from build123d import *

# Parameters (mm, degrees)
SKETCH1_W                        = 71
SKETCH1_H                        = 54
BOSS_EXTRUDE1_DEPTH              = 3.75
FILLET1_R                        = 1
SKETCH2_R                        = 7
CUT_EXTRUDE1_DEPTH               = 1
FILLET2_R                        = 0.25
SKETCH3_R                        = 0.5
CUT_EXTRUDE2_DEPTH               = 0.1
FILLET3_R                        = 0.25
M2_5_CLEARANCE_HOLE1_D           = 2.9
M2_5_CLEARANCE_HOLE1_DEPTH       = 1
M2_5_CLEARANCE_HOLE1_CSINK_D     = 2.95
M2_5_CLEARANCE_HOLE1_CSINK_ANGLE = 90
M2_5_CLEARANCE_HOLE1_TIP         = 0.871247898
M1_6_CLEARANCE_HOLE1_D           = 1


with BuildPart() as part:
    # Sketch1 → Boss-Extrude1 (new body)
    with BuildSketch(Plane.XY):
        Rectangle(SKETCH1_W, SKETCH1_H)
    extrude(amount=BOSS_EXTRUDE1_DEPTH)

    # Fillet1
    fillet1_edges = [part.edges().sort_by_distance(p)[0] for p in [
        (35.5, -27, 1.875),
        (-35.5, -27, 1.875),
        (-35.5, 27, 1.875),
        (35.5, 27, 1.875),
    ]]
    fillet(fillet1_edges, radius=FILLET1_R)

    # Sketch2 → Cut-Extrude1 (cut)
    with BuildSketch(Plane.XY.offset(3.75)):
        with BuildLine():
            Line((-34, -0.5), (-34, 17))
            Line((-34, 17), (-26.5, 24.5))
            Line((-26.5, 24.5), (-9, 24.5))
            ThreePointArc((-9, 24.5), (8.67766953, -18.17766953), (-34, -0.5))
        make_face()
        with Locations((-9, -0.5)):
            Circle(SKETCH2_R, mode=Mode.SUBTRACT)
    extrude(amount=-CUT_EXTRUDE1_DEPTH, mode=Mode.SUBTRACT)

    # Fillet2
    fillet2_edges = [part.edges().sort_by_distance(p)[0] for p in [
        (-16, -0.5, 3.75),
    ]]
    fillet(fillet2_edges, radius=FILLET2_R)

    # Sketch3 → Cut-Extrude2 (cut)
    with BuildSketch(Plane.XY.offset(3.75)):
        with Locations((-9, 4.1)):
            Circle(SKETCH3_R)
        with Locations((-12.983716857, 1.8)):
            Circle(SKETCH3_R)
        with Locations((-12.983716857, -2.8)):
            Circle(SKETCH3_R)
        with Locations((-9, -5.1)):
            Circle(SKETCH3_R)
        with Locations((-5.016283143, -2.8)):
            Circle(SKETCH3_R)
        with Locations((-5.016283143, 1.8)):
            Circle(SKETCH3_R)
    extrude(amount=-CUT_EXTRUDE2_DEPTH, mode=Mode.SUBTRACT)

    # Fillet3
    fillet3_edges = [part.edges().sort_by_distance(p)[0] for p in [
        (8.67766953, -18.17766953, 2.75),
        (-34, 8.25, 2.75),
        (-30.25, 20.75, 2.75),
        (-34, 17, 3.25),
        (-17.75, 24.5, 2.75),
        (-26.5, 24.5, 3.25),
        (-16, -0.5, 2.75),
        (8.67766953, -18.17766953, 3.75),
        (-17.75, 24.5, 3.75),
        (-30.25, 20.75, 3.75),
        (-34, 8.25, 3.75),
    ]]
    fillet(fillet3_edges, radius=FILLET3_R)

    # M2.5 Clearance Hole1
    with Locations(Plane.XY.offset(3.75)):
        with Locations((-9, -0.5)):
            CounterSinkHole(M2_5_CLEARANCE_HOLE1_D / 2, M2_5_CLEARANCE_HOLE1_CSINK_D / 2, depth=M2_5_CLEARANCE_HOLE1_DEPTH, counter_sink_angle=M2_5_CLEARANCE_HOLE1_CSINK_ANGLE)
            with Locations((0, 0, -(M2_5_CLEARANCE_HOLE1_DEPTH + M2_5_CLEARANCE_HOLE1_TIP / 2))):  # 118° drill point
                Cone(0, M2_5_CLEARANCE_HOLE1_D / 2, M2_5_CLEARANCE_HOLE1_TIP, mode=Mode.SUBTRACT)

    # M1.6 Clearance Hole1 (through all)
    with Locations(Plane.XY.offset(3.75)):
        with Locations((-169.780661566, 67.45785255), (-33.5, 22), (-30.6, 25), (3.1, 25), (33.5, 25), (8.2, 23.4), (33.5, -25), (3.1, -25), (-26.5, -21.5), (-29, -20), (-33.5, 25)):
            Hole(M1_6_CLEARANCE_HOLE1_D / 2)


solid = part.part
Design review of the part built by this model. Coordinates are the model's own, in mm. A direction names the side the tool comes from. Round coordinates to 2 decimals unless told otherwise and drop trailing zeros.
Item 1: For pin 1 Ø0.5 at (x, y) = (-13, 2) entering from +Z; pin 2 Ø8 at (x, y) = (-15.5, 19.5) entering from +Z, all flat-tipped, find the tip position at first contact; note any pin that passes through.
Item 2: For faces 1 (the cylindrical face through (-2.534, -3.181, 3.254)), 2 (the flat face through (0, 0, 0)), list the 3-axis set-ups (+Z, -Z, +X, -X, +Y, -Y) from which the entire face can be reached by the end or side of a thin tool; tool diameter is ignored.
Item 3: Wall thickness on L1, parallel to Y at x = 3, z = 1.35; L2, parallel to Y at x = -30.6, z = 1; L3, parallel to X at y = -1, z = 3.25 (3 decimals): over which ranges is each line inside the solid? List them lowest first.
Item 4: Draft analysis for pull direction Y (two halves, no side actions). For faces 3 (the cylindrical face through (-7.55, -0.44, 3.23)), 4 (the flat face through (23, 0, 3.75)), 5 (the flat face through (0, 27, 2)), state which applies: released by +Y, released by -Y, zero draft, split by the parting line, or undercut.
Check values:
1. pin 1: stops at z = 3.65
1. pin 2: stops at z = 2.75
2. face 1: +Z
2. face 2: -Z, +X, -X, +Y, -Y
3. L1: y = -27 to -25.49, -24.51 to 24.51, 25.49 to 27
3. L2: y = -27 to 24.5, 25.5 to 27
3. L3: x = -35.5 to -33.995, -15.982 to -10.361, -7.639 to -2.018, 15.995 to 35.5
4. face 3: undercut
4. face 4: zero draft
4. face 5: released by +Y
